from build123d import *

# Parameters (mm, degrees)
SKETCH_1_W          = 25
SKETCH_1_H          = 16
EXTRUDE_1_DEPTH     = 1
SKETCH_2_R          = 1.75
CUT_EXTRUDE_1_DEPTH = 2
SKETCH_3_R          = 2.5
SKETCH_3_R_2        = 1.5
EXTRUDE_2_DEPTH     = 12.5
FILLET_1_R          = 2


with BuildPart() as part:
    # 草图1 → 凸台-拉伸1 (new body)
    with BuildSketch(Plane(origin=(0, 0, 0), x_dir=(1, 0, 0), z_dir=(0, 1, 0))):
        Rectangle(SKETCH_1_W, SKETCH_1_H)
    extrude(amount=EXTRUDE_1_DEPTH)

    # 草图2 → 切除-拉伸1 (cut, through all)
    with BuildSketch(Plane(origin=(0, 1, 0), x_dir=(1, 0, 0), z_dir=(0, 1, 0))):
        with Locations((-7, -2.5)):
            Circle(SKETCH_2_R)
        with Locations((7, -2.5)):
            Circle(SKETCH_2_R)
    extrude(amount=-CUT_EXTRUDE_1_DEPTH, mode=Mode.SUBTRACT)

    # 草图3 → 凸台-拉伸2 (add)
    with BuildSketch(Plane(origin=(12.5, 0, 0), x_dir=(0, 0, -1), z_dir=(1, 0, 0))):
        with Locations((8, 2.5)):
            Circle(SKETCH_3_R)
        with Locations((8, 2.5)):
            Circle(SKETCH_3_R_2, mode=Mode.SUBTRACT)
    extrude(amount=-EXTRUDE_2_DEPTH)

    # 圆角1
    fillet_1_edges = [part.edges().sort_by_distance(p)[0] for p in [
        (12.5, 0.5, 8),
        (-12.5, 0.5, 8),
    ]]
    fillet(fillet_1_edges, radius=FILLET_1_R)


solid = part.part
For this review, take the finished solid that the model builds, in its own axes (mm). A direction names the side the tool comes from. Round coordinates to 2 decimals unless told otherwise and drop trailing zeros. Loops run counter-clockwise (first coordinate to the right, second up) from the corner with the lowest first, then second, coordinate; pieces in that order, holes last. Notation, with made-up numbers: (-31.75, 43) - (14.25, 43) arc R24 ccw to (14.25, 69) - close; hole circle Ø6 at (-35.75, 7.5). An arc over 180 degrees is marked (long way). Use one line per item in the form item = value.
Item 1: Consider section A-A on x = 7. Write out the cut boundary in (y, z), then the cut area to 3 significant figures.
Answers:
outline = (0, -8) arc R2.5 ccw (long way) to (1, -6) - (1, 0.75) - (0, 0.75) - close; (0, 4.25) - (1, 4.25) - (1, 8) - (0, 8) - close; hole circle Ø3 at (2.5, -8)
area = 23.7 mm^2
Item 2: Consider section C-C on z = 2.5. Write out the cut boundary in (x, y).
Answers:
outline = (-12.5, 0) - (-8.75, 0) - (-8.75, 1) - (-12.5, 1) - close; (-5.25, 0) - (5.25, 0) - (5.25, 1) - (-5.25, 1) - close; (8.75, 0) - (12.5, 0) - (12.5, 1) - (8.75, 1) - close
Item 3: Tool access review of faces 1 (the flat face through (-6.3, 0.5, -8)), 2 (the flat face through (-0.1, 0.5, 8)): name each direction out of +Z, -Z, +X, -X, +Y, -Y from which nothing blocks a thin tool from reaching the whole face with its end or side.
Answers:
face_1 = -Z, -X, +Y, -Y
face_2 = +Z, +X, -X, +Y, -Y
Item 4: Clearance check with flat-ended pins moving along their axes: P1, Ø1, axis at x = 6.5, z = -1, coming from the -Y side; P2, Ø1, axis at y = 3, z = 0, coming from the -X side; P3, Ø2, axis at x = -9, y = 1, coming from the -Z side. State where each tip first meets the part, or that it passes through.
Answers:
P1 = 0
P2 = through
P3 = -8
Item 5: Consider section D-D on x = -7. Write out the cut boundary in (y, z), then the cut area to 3 significant figures.
Answers:
outline = (0, -8) - (1, -8) - (1, 0.75) - (0, 0.75) - close; (0, 4.25) - (1, 4.25) - (1, 8) - (0, 8) - close
area = 12.5 mm^2
Item 6: For line 1 (X direction, y = 0.3, z = 2.5); line 2 (Z direction, x = -7, y = 0.7); line 3 (Y direction, x = -9.75, z = -6.5), list the stretches that pass through material, from the lowest coordinate up.
Answers:
line_1 = -12.5 to -8.75, -5.25 to 5.25, 8.75 to 12.5
line_2 = -8 to 0.75, 4.25 to 8
line_3 = 0 to 1
Item 7: Mouldability with a two-part tool opening along Z and no side actions: class faces 3 (the cylindrical face through (8.617, 0.507, 3.17)), 4 (the flat face through (0, 4, -9)), 5 (the cylindrical face through (-11.9, 0.51, 7.43)) as +Z half, -Z half, draft (parallel to the pull), parting line (faces both ways), or undercut.
Answers:
face_3 = undercut
face_4 = draft
face_5 = +Z half
Item 8: Consider section B-B on y = 2.5. Write out the cut boundary in (x, z), then the cut area to 3 significant figures.
Answers:
outline = (0, -10.5) - (12.5, -10.5) - (12.5, -9.5) - (0, -9.5) - close; (0, -6.5) - (12.5, -6.5) - (12.5, -5.5) - (0, -5.5) - close
area = 25.0 mm^2
